Build history of the part. All positions in model axes, mm. Give positions to 0.01 mm unless a question says otherwise; leave off trailing zeros. Loops run counter-clockwise (first coordinate to the right, second up) from the corner with the lowest first, then second, coordinate; pieces in that order, holes last. Notation, with made-up numbers: M -39.75,-39 L -0.75,-39 A33 ccw -0.75,-3 Z; hole C 0,-21 d7. An arc over 180 degrees is marked long. Answer in a Markdown table with one row per item. Add a question column.
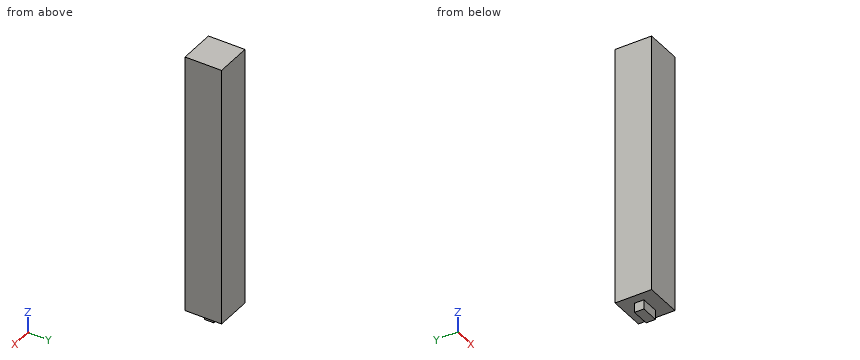
```python
from build123d import *

# Parameters (mm, degrees)
F0_W     = 3.5
F0_H     = 1.8
F1_DEPTH = 1.8
F2_W     = 7
F2_H     = 7
F2_W_2   = 3.5
F2_H_2   = 1.8
F3_DEPTH = 50


# Not quite as in the source:
# - a feature names something its author has since deleted; it is built from what else it names


with BuildPart() as f1:
    # F0 (on Front) → F1 (new body)
    with BuildSketch(Plane.XZ):
        with Locations((0, -25.45)):
            Rectangle(F0_W, F0_H)
    extrude(amount=F1_DEPTH)

    # F2 (on face) → F3 (join)
    with BuildSketch(Plane.XY.offset(-24.55)):
        with Locations((0, -0.9)):
            Rectangle(F2_W, F2_H)
        with Locations((0, -0.9)):
            Rectangle(F2_W_2, F2_H_2, mode=Mode.SUBTRACT)
        with Locations((0, -0.9)):
            Rectangle(F2_W_2, F2_H_2)
    extrude(amount=F3_DEPTH)


solid = f1.part
```
(1) Slice it at A-A, the plane x = 0.5. Give the cut face in (y, z), then the cut area to 3 significant figures.
(2) Wall check: line 1 (Z direction, x = -1.75, y = -2.25). Give the ranges that are in metal, low to high.
(3) Slice it at B-B, the plane y = -1. Give the cut face in (x, z), then the cut area to 3 significant figures.
(4) Slice it at D-D, the plane y = -3.5. Give the cut face in (x, z).
(5) Slice it at C-C, the plane x = 2.5. Give the cut face in (y, z), then the cut area to 3 significant figures.
(6) Pin check, flat tips, straight feed: pin 1 (0.5 mm diameter, centred on y = -1, z = -25.5, fed in from -X); pin 2 (0.5 mm diameter, centred on y = -1, z = -25.5, fed in from +X); pin 3 (0.9 mm diameter, centred on x = 1, z = -25.5, fed in from -Y). Stop position of each tip, or through.
Solution:
| question | item | result |
|---|---|---|
| 1 | outline | M -4.4,-24.55 L -1.8,-24.55 L -1.8,-26.35 L 0,-26.35 L 0,-24.55 L 2.6,-24.55 L 2.6,25.45 L -4.4,25.45 Z |
| 1 | area | 353 mm^2 |
| 2 | line 1 | -24.55 to 25.45 |
| 3 | outline | M -3.5,-24.55 L -1.75,-24.55 L -1.75,-26.35 L 1.75,-26.35 L 1.75,-24.55 L 3.5,-24.55 L 3.5,25.45 L -3.5,25.45 Z |
| 3 | area | 356 mm^2 |
| 4 | outline | M -3.5,-24.55 L 3.5,-24.55 L 3.5,25.45 L -3.5,25.45 Z |
| 5 | outline | M -4.4,-24.55 L 2.6,-24.55 L 2.6,25.45 L -4.4,25.45 Z |
| 5 | area | 350 mm^2 |
| 6 | pin 1 | x = -1.75 |
| 6 | pin 2 | x = 1.75 |
| 6 | pin 3 | y = -1.8 |
